Part model, mm, in its own coordinate system. Round coordinates to 2 decimals unless told otherwise and drop trailing zeros. Write each loop counter-clockwise with the first axis right and the second up, starting at its lowest first coordinate (ties: lowest second). Pieces come first, ordered by that corner, then holes. Notation, with made-up numbers: (14.5, -36) -> (43.5, -36) arc R33 ccw to (43.5, -3) -> close; hole circle Ø6 at (-9.75, 36.25). An arc over 180 degrees is marked (long way). Return JSON: item names as keys, results as strings. Group by question number.
(1) Drill centre lines: L1, parallel to X at y = 0, z = -0.1; L2, parallel to X at y = -55, z = 0.25; L3, parallel to Y at x = 68, z = -0.4. Where is each one in solid material? Low to high. Write a range as from..to.
(2) Saw through at D-D (x = 52.5). List the corners of the cut face in (y, z), plus the area to 3 significant figures.
(3) Saw through at B-B (x = -68). List the corners of the cut face in (y, z), plus the area to 3 significant figures.
(4) Saw through at A-A (z = 0.15). State how many separate pieces and enclosed holes the cut face has, plus the area to 3 significant figures.
(5) Mould opens along X. For faces 1 (the flat face through (2, 25, 1)), 2 (the cylindrical face through (119.884, -5.276, -0.479)), 3 (the cylindrical face through (-65.8, 51.6, -0.5)) say: +X half, -X half, draft (parallel to the pull), parting line (faces both ways), or undercut.
(6) Drop flat-ended pins along their axis: pin 1 Ø1 at (y, z) = (-68.5, 0) entering from +X; pin 2 Ø1 at (y, z) = (74, -1.5) entering from -X; pin 3 Ø1 at (y, z) = (-67, -1.5) entering from +X. Give the stop position or say it passes through.
(7) Saw through at C-C (y = 67.5). List the corners of the cut face in (x, z).
Autodesk Fusion 360 part; units mm, degrees
sketch "スケッチ1" plane through (0, 0, 0) normal (0, 0, 1) x (1, 0, 0)
  line L0 (68, -55) -> (-68, -55)
  line L1 (-68, -55) -> (-68, 55)
  line L2 (-68, 55) -> (68, 55)
  line L3 (68, 55) -> (68, -55)
  line L4 (68, -55) -> (-68, 55) construction
  line L5 (-68, -55) -> (68, 55) construction
  circle A0 centre (-68, 55) radius 4.05
  circle A1 centre (68, 55) radius 4.05
  circle A2 centre (-68, -55) radius 4.05
  circle A3 centre (68, -55) radius 4.05
  circle A4 centre (0, 0) radius 35
  circle A5 centre (0, 0) radius 130
  dimension "d1" = 136
  dimension "d2" = 110
  dimension "d3" = 8.1
  dimension "d4" = 8.1
  dimension "d5" = 8.1
  dimension "d6" = 8.1
  dimension "d18" = 70
  dimension "d19" = 260
extrude "押し出し1" add sketch "スケッチ1" along normal blind 1 contours L0 L1 L2 L3 A0 A1 A2 A3 | A5
sketch "スケッチ7" plane through (0, 0, 1) normal (0, 0, 1) x (-1, 0, 0)
  circle A0 centre (68, -55) radius 4.05
  circle A1 centre (68, 55) radius 4.05
  circle A2 centre (-68, -55) radius 4.05
  circle A3 centre (-68, 55) radius 4.05
  circle A4 centre (0, 0) radius 35
  circle A5 centre (0, 0) radius 130
  circle A6 centre (0, 0) radius 25
  dimension "d809" = 50
extrude "押し出し11" add sketch "スケッチ7" against normal blind 1 contours A4
sketch "スケッチ8" plane through (0, 0, 1) normal (0, 0, 1) x (-1, 0, 0)
  circle A0 centre (0, 0) radius 25
  circle A1 centre (68, -55) radius 4.05
  circle A2 centre (68, 55) radius 4.05
  circle A3 centre (-68, -55) radius 4.05
  circle A4 centre (-68, 55) radius 4.05
  circle A5 centre (0, 0) radius 130
  line L0 (0, 0) -> (16.5, 0)
  line L1 (16.5, 0) -> (16.5, 25.6)
  circle A6 centre (16.5, 25.6) radius 1.25
  line L2 (0, 0) -> (-16.5, 0)
  line L3 (-16.5, 0) -> (-16.5, -25.6)
  circle A7 centre (-16.5, -25.6) radius 1.25
  line L4 (-16.5, -25.6) -> (-37.5, -25.6)
  circle A8 centre (-37.5, -25.6) radius 1.25
  line L5 (-27, -25.6) -> (-27, -36.1)
  line L6 (-27, -25.6) -> (-27, -15.1)
  circle A9 centre (-27, -36.1) radius 1.25
  circle A10 centre (-27, -15.1) radius 1.25
  dimension "d812" = 16.5
  dimension "d813" = 25.6
  dimension "d814" = 2.5
  dimension "d817" = 16.5
  dimension "d818" = 25.6
  dimension "d819" = 2.5
  dimension "d822" = 21
  dimension "d823" = 2.5
  dimension "d824" = 10.5
  dimension "d825" = 10.5
  dimension "d826" = 2.5
  dimension "d827" = 2.5
extrude "押し出し13" cut sketch "スケッチ8" against normal blind 1 contours A9 | A8 | A10 | L3 A7 L4 | L3 A7 L4
sketch "スケッチ9" plane through (0, 0, 1) normal (0, 0, 1) x (-1, 0, 0)
  circle A0 centre (-27, -36.1) radius 1.25
  circle A1 centre (-37.5, -25.6) radius 1.25
  circle A2 centre (-16.5, -25.6) radius 1.25
  circle A3 centre (-27, -15.1) radius 1.25
  circle A4 centre (0, 0) radius 25
  circle A5 centre (68, -55) radius 4.05
  circle A6 centre (68, 55) radius 4.05
  circle A7 centre (-68, -55) radius 4.05
  circle A8 centre (-68, 55) radius 4.05
  circle A9 centre (0, 0) radius 130
  circle A10 centre (0, 0) radius 120
  dimension "d828" = -10
extrude "押し出し14" cut sketch "スケッチ9" against normal blind 1 contours A9
sketch "スケッチ10" plane through (0, 0, 1) normal (0, 0, 1) x (-1, 0, 0)
  circle A0 centre (0, 0) radius 120
  circle A1 centre (-27, -36.1) radius 1.25
  circle A2 centre (-37.5, -25.6) radius 1.25
  circle A3 centre (-16.5, -25.6) radius 1.25
  circle A4 centre (-27, -15.1) radius 1.25
  circle A5 centre (0, 0) radius 25
  circle A6 centre (68, -55) radius 4.05
  circle A7 centre (68, 55) radius 4.05
  circle A8 centre (-68, -55) radius 4.05
  circle A9 centre (-68, 55) radius 4.05
  line L0 (0, 0) -> (0, 40)
  line L1 (0, 40) -> (-15, 40)
  line L2 (0, 40) -> (15, 40)
  circle A10 centre (15, 40) radius 1.25
  circle A11 centre (-15, 40) radius 1.25
  dimension "d838" = 40
  dimension "d839" = 15
  dimension "d840" = 15
  dimension "d841" = 2.5
  dimension "d842" = 2.5
extrude "押し出し16" cut sketch "スケッチ10" against normal blind 1 contours A11 | A10
sketch "スケッチ11" plane through (0, 0, 1) normal (0, 0, 1) x (-1, 0, 0)
  circle A0 centre (-15, 40) radius 1.25
  circle A1 centre (15, 40) radius 1.25
  circle A2 centre (0, 0) radius 120
  circle A3 centre (-27, -36.1) radius 1.25
  circle A4 centre (-37.5, -25.6) radius 1.25
  circle A5 centre (-16.5, -25.6) radius 1.25
  circle A6 centre (-27, -15.1) radius 1.25
  circle A7 centre (0, 0) radius 25
  circle A8 centre (68, -55) radius 4.05
  circle A9 centre (68, 55) radius 4.05
  circle A10 centre (-68, -55) radius 4.05
  circle A11 centre (-68, 55) radius 4.05
  line L0 (0, 0) -> (0, 107)
  line L1 (0, 107) -> (15, 107)
  line L2 (0, 107) -> (-15, 107)
  circle A12 centre (15, 107) radius 1.25
  circle A13 centre (-15, 107) radius 1.25
  dimension "d845" = 107
  dimension "d846" = 15
  dimension "d847" = 15
  dimension "d848" = 2.5
  dimension "d849" = 2.5
extrude "押し出し17" cut sketch "スケッチ11" against normal blind 1 contours A13 | A12
sketch "スケッチ12" plane through (0, 0, 1) normal (0, 0, 1) x (-1, 0, 0)
  circle A0 centre (15, 107) radius 1.25
  circle A1 centre (-15, 107) radius 1.25
  circle A2 centre (-15, 40) radius 1.25
  circle A3 centre (15, 40) radius 1.25
  circle A4 centre (0, 0) radius 120
  circle A5 centre (-27, -36.1) radius 1.25
  circle A6 centre (-37.5, -25.6) radius 1.25
  circle A7 centre (-16.5, -25.6) radius 1.25
  circle A8 centre (-27, -15.1) radius 1.25
  circle A9 centre (0, 0) radius 25
  circle A10 centre (68, -55) radius 4.05
  circle A11 centre (68, 55) radius 4.05
  circle A12 centre (-68, -55) radius 4.05
  circle A13 centre (-68, 55) radius 4.05
  line L0 (-37.5, -25.6) -> (-37.5, 0)
  circle A14 centre (-37.5, 0) radius 1.25
  line L1 (-27, -15.1) -> (-27, 10.5)
  circle A15 centre (-27, 10.5) radius 1.25
  line L2 (-27, -36.1) -> (-27, -10.5)
  circle A16 centre (-27, -10.5) radius 1.25
  dimension "d852" = 25.6
  dimension "d853" = 2.5
  dimension "d854" = 25.6
  dimension "d855" = 2.5
  dimension "d856" = 25.6
  dimension "d857" = 2.5
extrude "押し出し18" add sketch "スケッチ12" against normal blind 1 contours A5 | A8 L1 L2 | A8 L1 L2 | A6 | A7
extrude "押し出し19" cut sketch "スケッチ12" against normal blind 1 contours A15 | L1 L2 A16 | L1 L2 A16 | A14
extrude "押し出し20" add 1 faces at (-71.1115, 16.9879, 0) along direction (0, 0, -1) blind 2
sketch "スケッチ13" plane through (0, 0, 1) normal (0, 0, 1) x (-1, 0, 0)
  circle A0 centre (-37.5, 0) radius 1.25
  circle A1 centre (-27, 10.5) radius 1.25
  circle A2 centre (-27, -10.5) radius 1.25
  circle A3 centre (15, 107) radius 1.25
  circle A4 centre (-15, 107) radius 1.25
  circle A5 centre (-15, 40) radius 1.25
  circle A6 centre (15, 40) radius 1.25
  circle A7 centre (0, 0) radius 120
  circle A8 centre (0, 0) radius 25
  circle A9 centre (68, -55) radius 4.05
  circle A10 centre (68, 55) radius 4.05
  circle A11 centre (-68, -55) radius 4.05
  circle A12 centre (-68, 55) radius 4.05
  circle A13 centre (0, 0) radius 20
  dimension "d864" = 40
extrude "押し出し21" add sketch "スケッチ13" against normal blind 3 contours A8
sketch "スケッチ14" plane through (0, 0, 1) normal (0, 0, 1) x (-1, 0, 0)
  circle A0 centre (0, 0) radius 20
  circle A1 centre (-37.5, 0) radius 1.25
  circle A2 centre (-27, 10.5) radius 1.25
  circle A3 centre (-27, -10.5) radius 1.25
  circle A4 centre (15, 107) radius 1.25
  circle A5 centre (-15, 107) radius 1.25
  circle A6 centre (-15, 40) radius 1.25
  circle A7 centre (15, 40) radius 1.25
  circle A8 centre (0, 0) radius 120
  circle A9 centre (68, -55) radius 4.05
  circle A10 centre (68, 55) radius 4.05
  circle A11 centre (-68, -55) radius 4.05
  circle A12 centre (-68, 55) radius 4.05
  line L0 (-37.5, 0) -> (-37, 0)
  line L1 (-27, -10.5) -> (-26.5, -10.5)
  line L2 (-27, 10.5) -> (-26.5, 10.5)
  circle A13 centre (-26.5, -10.5) radius 1.25
  circle A14 centre (-37, 0) radius 1.25
  circle A15 centre (-26.5, 10.5) radius 1.25
  dimension "d867" = 0.5
  dimension "d868" = 0.5
  dimension "d869" = 0.5
  dimension "d870" = 2.5
  dimension "d871" = 2.5
  dimension "d872" = 2.5
extrude "押し出し22" cut sketch "スケッチ14" against normal blind 3 contours A1 A14 | A2 A15 | A3 A13 picked at (-35.9431, -0.2395) picked at (-25.4431, 10.2605) picked at (-25.4431, -10.7395)
extrude "押し出し23" add sketch "スケッチ14" against normal blind 3 contours A1 A14 | A2 A15 | A3 A13 picked at (-35.9431, -0.2395) picked at (-25.4431, 10.2605) picked at (-25.4431, -10.7395)
sketch "スケッチ15" plane through (0, 0, 1) normal (0, 0, 1) x (-1, 0, 0)
  circle A0 centre (-68, 55) radius 4.05
  circle A1 centre (-68, -55) radius 4.05
  circle A2 centre (68, 55) radius 4.05
  circle A3 centre (68, -55) radius 4.05
  circle A4 centre (0, 0) radius 120
  circle A5 centre (15, 40) radius 1.25
  circle A6 centre (-15, 40) radius 1.25
  circle A7 centre (-15, 107) radius 1.25
  circle A8 centre (15, 107) radius 1.25
  circle A9 centre (-26.5, -10.5) radius 1.25
  circle A10 centre (-26.5, 10.5) radius 1.25
  circle A11 centre (-37, 0) radius 1.25
  circle A12 centre (0, 0) radius 20
  circle A13 centre (0, 0) radius 19.5
  dimension "d877" = 39
extrude "押し出し24" add sketch "スケッチ15" against normal blind 3 contours A12
Computed values:
{
 "1": {"L1": "-120..-19.5, 19.5..36.25, 38.75..120", "L2": "-106.65..-72.05, -63.95..63.95, 72.05..106.65", "L3": "-98.87..-59.05, -50.95..50.95, 59.05..98.87"},
 "2": {"outline": "(-107.91, -2) -> (107.91, -2) -> (107.91, 1) -> (-107.91, 1) -> close", "area": "647 mm2"},
 "3": {"outline": "(-98.87, -2) -> (-59.05, -2) -> (-59.05, 1) -> (-98.87, 1) -> close; (-50.95, -2) -> (50.95, -2) -> (50.95, 1) -> (-50.95, 1) -> close; (59.05, -2) -> (98.87, -2) -> (98.87, 1) -> (59.05, 1) -> close", "area": "545 mm2"},
 "4": {"separate pieces": "1", "enclosed holes": "12", "area": "43,800 mm2"},
 "5": {"face 1": "draft", "face 2": "parting line", "face 3": "undercut"},
 "6": {"pin 1": "x = 98.87", "pin 2": "x = -94.86", "pin 3": "x = 99.89"},
 "7": {"outline": "(-99.22, -2) -> (99.22, -2) -> (99.22, 1) -> (-99.22, 1) -> close"}
}
